```python
from build123d import *

# Parameters (mm, degrees)
EXTRUDE_1_DEPTH     = 3
SKETCH_3_R          = 7
CUT_EXTRUDE_1_DEPTH = 64.576725301
SKETCH_4_R          = 1
CUT_EXTRUDE_2_DEPTH = 64.576725301
SKETCH_5_R          = 2
EXTRUDE_2_DEPTH     = 3
FILLET_1_RADIUS     = 5
FILLET_1_LENGTH     = 3
SKETCH_6_R          = 1.85
CUT_EXTRUDE_3_DEPTH = 1.5


with BuildPart() as part:
    # 草图1 → 凸台-拉伸1 (new body)
    with BuildSketch(Plane.XY):
        Polygon((-18, 0), (18, 0), (18, 5), (-12.022213998, 57), (-28, 57), (-28, 47), (-18, 47), align=None)
    extrude(amount=EXTRUDE_1_DEPTH)

    # 草图3 → 切除-拉伸1 (cut, through all)
    with BuildSketch(Plane.XY.offset(3)):
        with Locations((-6.476357534, 13.687539211)):
            Circle(SKETCH_3_R)
    extrude(amount=-CUT_EXTRUDE_1_DEPTH, mode=Mode.SUBTRACT)

    # 草图4 → 切除-拉伸2 (cut, through all)
    with BuildSketch(Plane.XY.offset(3)):
        with Locations((12, 2.5)):
            Circle(SKETCH_4_R)
        with Locations(Location((-12, 2.5, 0), (0, 0, 180))):
            Circle(SKETCH_4_R)
    extrude(amount=-CUT_EXTRUDE_2_DEPTH, mode=Mode.SUBTRACT)

    # 草图5 → 凸台-拉伸2 (add)
    with BuildSketch(Plane.XY.offset(3)):
        with Locations(Location((-23, 52, 0), (0, 0, 180))):
            Circle(SKETCH_5_R)
    extrude(amount=EXTRUDE_2_DEPTH)

    # 圆角1: full round fillet: the end face becomes a half cylinder, R = half its width
    fillet_1_face = Plane((-28, 52, 1.5), x_dir=(0, 0, 1), z_dir=(-1, 0, 0))  # on the end face: x along it, z out of the body
    fillet_1_slab = fillet_1_face.offset(-FILLET_1_RADIUS / 2) * Box(FILLET_1_LENGTH, 2 * FILLET_1_RADIUS, FILLET_1_RADIUS, mode=Mode.PRIVATE)  # the body's end, R deep
    fillet_1_round = Plane((-23, 52, 1.5), x_dir=(-1, 0, 0), z_dir=(0, 0, 1)) * Cylinder(FILLET_1_RADIUS, FILLET_1_LENGTH, mode=Mode.PRIVATE)  # its axis R under the face
    add(fillet_1_slab - fillet_1_round, mode=Mode.SUBTRACT)

    # 草图6 → 切除-拉伸3 (cut)
    with BuildSketch(Plane.XY.offset(3)):
        with Locations((12, 2.5)):
            Circle(SKETCH_6_R)
        with Locations((-12, 2.5)):
            Circle(SKETCH_6_R)
    extrude(amount=-CUT_EXTRUDE_3_DEPTH, mode=Mode.SUBTRACT)


solid = part.part
```
Could you check a few things on this model? Use its own coordinates, in mm. A direction names the side the tool comes from. Give positions to 0.01 mm unless a question says otherwise; leave off trailing zeros. Order: outer loops, then holes, each group sorted by start corner. A loop starts at its lowest first (then second) coordinate and runs counter-clockwise, first axis right, second up.
Q1. Suppose I cut it at A-A, the plane x = -2.5. Write out the boundary of the cut face in (y, z), and give its area (3 significant figures).
Q2. If I drill on line 1 along Y through (x, z) = (-12, 0.6); line 2 along Z through (x, y) = (15, 3); line 3 along Y through (x, z) = (12, 0.4), over which ranges is the centre line in solid material (lowest first)?
Q3. Suppose I cut it at C-C, the plane z = 0.75. Write out the boundary of the cut face in (x, y).
Q4. I'm going to push flat-ended pins straight in: P1, Ø4, axis at x = 12.5, y = 3, coming from the +Z side; P2, Ø1.6, axis at x = 12, y = 2.5, coming from the +Z side (3 decimals); P3, Ø3, axis at y = 44, z = 2.5, coming from the +X side; P4, Ø0.9, axis at y = 29, z = 1.5, coming from the -X side. Where does each tip first touch, or does it pass through?
Q5. We'd pull the mould along Y, two halves only. Please class faces 4 (the cylindrical face through (13.765, 3.056, 2.26)), 5 (the cylindrical face through (-28, 52, 2)), 6 (the flat face through (-18, 24, 1)), 7 (the flat face through (0, 0, 1)): +Y half, -Y half, draft (parallel to the pull), parting line (faces both ways), or undercut.
Q6. Suppose I cut it at B-B, the plane y = 15.5. Write out the boundary of the cut face in (x, z), and give its area (3 significant figures).
Q7. Suppose I cut it at D-D, the plane x = 12. Write out the boundary of the cut face in (y, z).
Q8. For faces 1 (the cylindrical face through (-10.235, 3.056, 2.26)), 2 (the cylindrical face through (-11.2, 3.1, 0.8)), 3 (the flat face through (-21, 47, 1)), which set-ups out of +Z, -Z, +X, -X, +Y, -Y let a thin tool reach every point of the face, with its end or its side?
Solution:
1. outline: (0, 0) - (7.93, 0) - (7.93, 3) - (0, 3) - close; (19.45, 0) - (40.51, 0) - (40.51, 3) - (19.45, 3) - close
1. area: 87.0 mm2
2. line 1: y = 0 to 1.5, 3.5 to 9.39, 17.99 to 56.96
2. line 2: z = 0 to 3
2. line 3: y = 0 to 1.5, 3.5 to 15.39
3. outline: (-23, 47) - (-18, 47) - (-18, 0) - (18, 0) - (18, 5) - (-12.02, 57) - (-23, 57) arc R5 ccw to start; hole circle Ø14 at (-6.48, 13.69); hole circle Ø2 at (-12, 2.5); hole circle Ø2 at (12, 2.5)
4. P1: stops at z = 3
4. P2: passes through
4. P3: stops at x = -3.65
4. P4: stops at x = -18
5. face 4: undercut
5. face 5: parting line
5. face 6: draft
5. face 7: -Y half
6. outline: (-18, 0) - (-13.24, 0) - (-13.24, 3) - (-18, 3) - close; (0.28, 0) - (11.94, 0) - (11.94, 3) - (0.28, 3) - close
6. area: 49.2 mm2
7. outline: (0, 0) - (1.5, 0) - (1.5, 1.5) - (0.65, 1.5) - (0.65, 3) - (0, 3) - close; (3.5, 0) - (15.39, 0) - (15.39, 3) - (4.35, 3) - (4.35, 1.5) - (3.5, 1.5) - close
8. face 1: +Z
8. face 2: +Z, -Z
8. face 3: +Z, -Z, -X, -Y
